from build123d import *

# Parameters (mm, degrees)
F0_R     = 5
F1_DEPTH = 25
F2_R     = 2
F3_R     = 1


with BuildPart() as f1:
    # F0 (on Top) → F1 (new body)
    with BuildSketch(Plane.XY):
        Polygon((0, 28.313708), (0, 0), (28.313708, 0), align=None)
        with Locations((9, 8)):
            Circle(F0_R, mode=Mode.SUBTRACT)
    extrude(amount=F1_DEPTH)

    # F2
    f2_edges = [f1.edges().sort_by_distance(p)[0] for p in [
        (0, 28.313708, 12.5),
        (28.313708, 0, 12.5),
    ]]
    fillet(f2_edges, radius=F2_R)

    # F3
    f3_edges = [f1.edges().sort_by_distance(p)[0] for p in [
        (14, 8, 12.5),
        (4, 8, 0),
        (4, 8, 25),
    ]]
    fillet(f3_edges, radius=F3_R)


solid = f1.part
The listing builds one solid part. Answer for the finished solid, in the listing's coordinates (mm). Coordinates: 2 decimals unless noted, no trailing zeros. Loops run counter-clockwise (first coordinate to the right, second up) from the corner with the lowest first, then second, coordinate; pieces in that order, holes last. Notation, with made-up numbers: (66, -7) -> (116, -7) arc R13 ccw to (116, 17) -> close; hole circle Ø8 at (-9.5, -24). An arc over 180 degrees is marked (long way). Answer in a Markdown table with one row per item. Add a question column.
1. Consider line 1 (Y direction, x = 9, z = 17.25); line 2 (Y direction, x = 13, z = 15.5); line 3 (X direction, y = 8.5, z = 13). Determine where each line is inside the solid, lowest interval first. Write a range as [from, to].
2. Determine the mould class of faces 1 (the flat face through (13, 13, 25)), 2 (the flat face through (12, 0, 12)), 3 (the cylindrical face through (1.2, 25.32, 12.68)), 4 (the cylindrical face through (13.77, 9.5, 12.34)) for opening direction Y: +Y half, -Y half, draft (parallel to the pull), parting line (faces both ways), or undercut.
3. The part is cut by section B-B, the plane z = 10.5. Write down the section's boundary in (x, y), then the cut area to 3 significant figures.
4. The part is cut by section D-D, the plane x = 18.75. Write down the section's boundary in (y, z), then the cut area to 3 significant figures.
5. Flat-ended cylindrical pins translate along their axes: P1, Ø8, axis at x = 9, y = 8, coming from the +Z side; P2, Ø6, axis at x = 21, y = 11, coming from the -Z side; P3, Ø3, axis at x = 15, z = 19, coming from the +Y side; P4, Ø3, axis at x = 14.5, z = 12.5, coming from the +Y side. Find the tip coordinate at first contact, or state that the pin passes through.
6. The part is cut by section A-A, the plane y = 8. Write down the section's boundary in (x, z).
7. The part is cut by section C-C, the plane x = 9. Write down the section's boundary in (y, z), then the cut area to 3 significant figures.
Answer below:
| question | item | result |
|---|---|---|
| 1 | line 1 | [0, 3], [13, 19.31] |
| 1 | line 2 | [0, 5], [11, 15.31] |
| 1 | line 3 | [0, 4.03], [13.97, 19.81] |
| 2 | face 1 | draft |
| 2 | face 2 | -Y half |
| 2 | face 3 | +Y half |
| 2 | face 4 | undercut |
| 3 | outline | (0, 0) -> (23.49, 0) arc R2 ccw to (24.9, 3.41) -> (3.41, 24.9) arc R2 ccw to (0, 23.49) -> close; hole circle Ø10 at (9, 8) |
| 3 | area | 312 mm2 |
| 4 | outline | (0, 0) -> (9.56, 0) -> (9.56, 25) -> (0, 25) -> close |
| 4 | area | 239 mm2 |
| 5 | P1 | through |
| 5 | P2 | z = 0 |
| 5 | P3 | y = 14.81 |
| 5 | P4 | y = 15.31 |
| 6 | outline | (0, 0) -> (3, 0) arc R1 ccw to (4, 1) -> (4, 24) arc R1 ccw to (3, 25) -> (0, 25) -> close; (14, 1) arc R1 ccw to (15, 0) -> (20.31, 0) -> (20.31, 25) -> (15, 25) arc R1 ccw to (14, 24) -> close |
| 7 | outline | (0, 0) -> (2, 0) arc R1 ccw to (3, 1) -> (3, 24) arc R1 ccw to (2, 25) -> (0, 25) -> close; (13, 1) arc R1 ccw to (14, 0) -> (19.31, 0) -> (19.31, 25) -> (14, 25) arc R1 ccw to (13, 24) -> close |
| 7 | area | 232 mm2 |
